For this review, use the dimensioned drawing (mm, ordinates from the lowest corner) and the shaded views. A direction names the side the tool comes from. Round coordinates to 2 decimals unless told otherwise and drop trailing zeros. Order: outer loops, then holes, each group sorted by start corner. A loop starts at its lowest first (then second) coordinate and runs counter-clockwise, first axis right, second up. Notation, with made-up numbers: (-27.75, -21.75) -> (10.25, -21.75) arc R20 ccw to (10.25, -4.75) -> close; hole circle Ø2 at (17, 22). An arc over 180 degrees is marked (long way). Use a Markdown table: item, result. Add a question column.
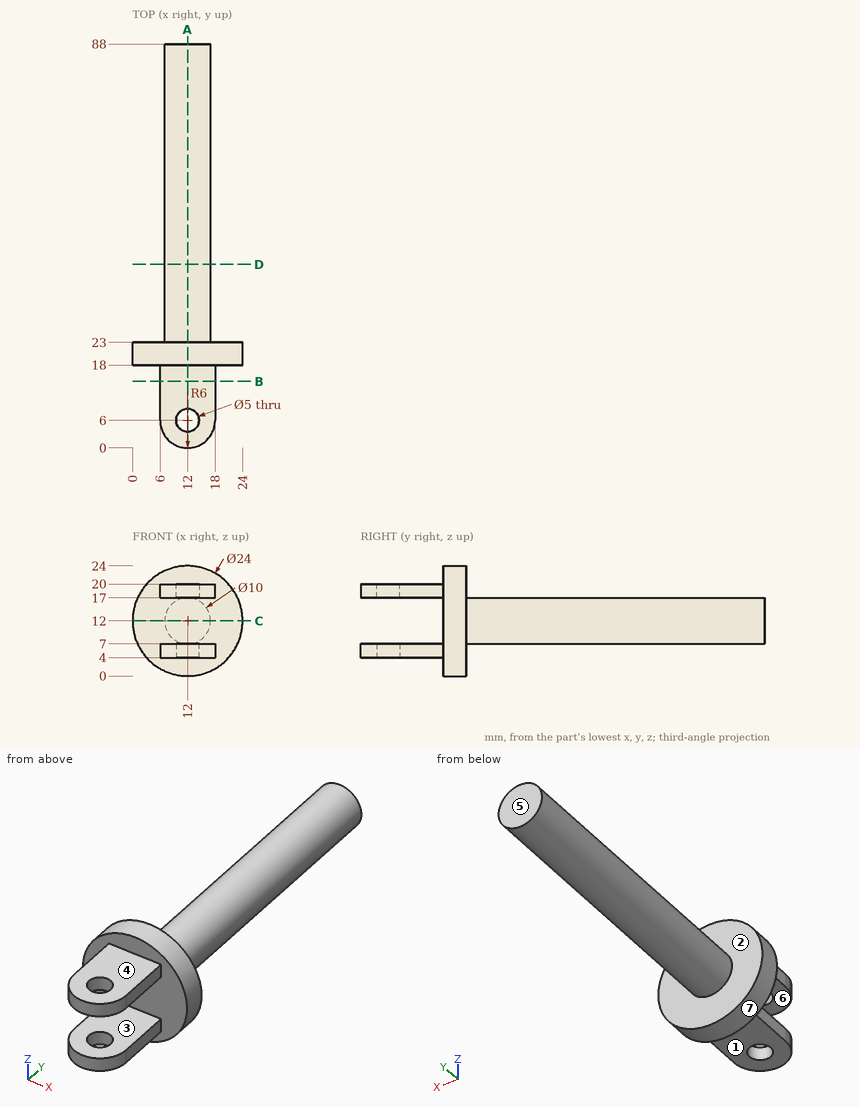
Q1. Insertion check: pin 1 (3.5 mm diameter, centred on x = 13, y = 13, fed in from +Z); pin 2 (3 mm diameter, centred on x = 14, z = 4.5, fed in from +Y); pin 3 (1 mm diameter, centred on x = 11.5, z = 2.5, fed in from -Y). Each pin has a flat end and moves straight along its axis. Give the tip position at first contact, or say it passes through.
Q2. Add section C-C (z = 12). Write out the cut boundary in (x, y), then the cut area to 3 significant figures.
Q3. Machinability: for the marked faces 1, 2, 3 and 4, which of the approach directions +Z, -Z, +X, -X, +Y, -Y give a long, thin tool a straight path to every point of the face, cutting with its end or side? Answer none if there is none.
Q4. Mouldability with a two-part tool opening along Z and no side actions: class the marked faces 5, 6 and 7 as pulls with the +Z half, pulls with the -Z half, needs draft (parallel to the pull), parting line crosses it, or undercut.
Q5. Add section A-A (x = 12). Write out the cut boundary in (y, z), then the cut area to 3 significant figures.
Q6. Wall thickness on line 1 (X direction, y = 6, z = 6.45); line 2 (Z direction, x = 11.5, y = 14.5); line 3 (Y direction, x = 12, z = 5.1): over which ranges is each line inside the solid? List them lowest first. Write a range as [from, to].
Q7. Add section B-B (y = 14.5). Write out the cut boundary in (x, z), then the cut area to 3 significant figures.
Q8. Add section D-D (y = 40). Write out the cut boundary in (x, z), then the cut area to 3 significant figures.
Report:
| question | item | result |
|---|---|---|
| 1 | pin 1 | stops at z = 20 |
| 1 | pin 2 | stops at y = 23 |
| 1 | pin 3 | stops at y = 18 |
| 2 | outline | (0, 18) -> (24, 18) -> (24, 23) -> (17, 23) -> (17, 88) -> (7, 88) -> (7, 23) -> (0, 23) -> close |
| 2 | area | 770 mm² |
| 3 | face 1 | -Z, +X, -X, -Y |
| 3 | face 2 | +Y |
| 3 | face 3 | +X, -X, -Y |
| 3 | face 4 | +Z, +X, -X, -Y |
| 4 | face 5 | needs draft |
| 4 | face 6 | undercut |
| 4 | face 7 | parting line crosses it |
| 5 | outline | (0, 4) -> (3.5, 4) -> (3.5, 7) -> (0, 7) -> close; (0, 17) -> (3.5, 17) -> (3.5, 20) -> (0, 20) -> close; (8.5, 4) -> (18, 4) -> (18, 0) -> (23, 0) -> (23, 7) -> (88, 7) -> (88, 17) -> (23, 17) -> (23, 24) -> (18, 24) -> (18, 20) -> (8.5, 20) -> (8.5, 17) -> (18, 17) -> (18, 7) -> (8.5, 7) -> close |
| 5 | area | 848 mm² |
| 6 | line 1 | x = [6, 9.5], [14.5, 18] |
| 6 | line 2 | z = [4, 7], [17, 20] |
| 6 | line 3 | y = [0, 3.5], [8.5, 23] |
| 7 | outline | (6, 4) -> (18, 4) -> (18, 7) -> (6, 7) -> close; (6, 17) -> (18, 17) -> (18, 20) -> (6, 20) -> close |
| 7 | area | 72.0 mm² |
| 8 | outline | circle Ø10 at (12, 12) |
| 8 | area | 78.5 mm² |
